Work out the finished part from the listing and answer in its coordinate system (mm). Face numbers are marked on the shaded views. A direction names the side the tool comes from. Give positions to 0.01 mm unless a question says otherwise; leave off trailing zeros. Loops run counter-clockwise (first coordinate to the right, second up) from the corner with the lowest first, then second, coordinate; pieces in that order, holes last. Notation, with made-up numbers: (-20.5, -39) - (30.5, -39) arc R22 cw to (30.5, -31) - close; hole circle Ø2 at (61, 75.25). An arc over 180 degrees is marked (long way). Use CSV: the item, a comma, the result in double quotes.
from build123d import *

# Parameters (mm, degrees)
F0_W     = 10
F0_H     = 10
F0_R     = 1.65
F1_DEPTH = 6
F0_R_2   = 4.65
F2_DEPTH = 2
F3_SIZE  = 2


with BuildPart() as f1:
    # F0 (on Top) → F1 (new body)
    with BuildSketch(Plane.XY):
        with Locations((0, 7.5)):
            Rectangle(F0_W, F0_H)
        with Locations((0, 7.5)):
            Circle(F0_R, mode=Mode.SUBTRACT)
    extrude(amount=F1_DEPTH)



with BuildPart() as f1b:
    # F0 (on Top) → F1, piece 2 (new body)
    with BuildSketch(Plane.XY):
        with Locations((0, -7.5)):
            Rectangle(F0_W, F0_H)
        with Locations((0, -7.5)):
            Circle(F0_R, mode=Mode.SUBTRACT)
    extrude(amount=F1_DEPTH)


with BuildPart() as f1_1:
    add(f1.part)

    add(f1b.part)  # F2 merges F1b
    # F0 (on Top) → F2 (join)
    with BuildSketch(Plane.XY):
        with BuildLine():
            Line((20, 25), (-20, 25))
            ThreePointArc((-20, 25), (-23.5355339059, 23.5355339059), (-25, 20))
            Line((-25, 20), (-25, -20))
            ThreePointArc((-25, -20), (-23.5355339059, -23.5355339059), (-20, -25))
            Line((-20, -25), (20, -25))
            ThreePointArc((20, -25), (23.5355339059, -23.5355339059), (25, -20))
            Line((25, -20), (25, 20))
            ThreePointArc((25, 20), (23.5355339059, 23.5355339059), (20, 25))
        make_face()
        with Locations((-17.9289321881, -17.9289321881)):
            Circle(F0_R_2, mode=Mode.SUBTRACT)
        with Locations((17.9289321881, -17.9289321881)):
            Circle(F0_R_2, mode=Mode.SUBTRACT)
        with Locations((0, -7.5)):
            Rectangle(F0_W, F0_H, mode=Mode.SUBTRACT)
        with Locations((-17.9289321881, 17.9289321881)):
            Circle(F0_R_2, mode=Mode.SUBTRACT)
        with Locations((0, 7.5)):
            Rectangle(F0_W, F0_H, mode=Mode.SUBTRACT)
        with Locations((17.9289321881, 17.9289321881)):
            Circle(F0_R_2, mode=Mode.SUBTRACT)
    extrude(amount=F2_DEPTH)

    # F3
    f3_edges = [f1_1.edges().sort_by_distance(p)[0] for p in [
        (0, -12.5, 2),
        (5, -7.5, 2),
        (5, 7.5, 2),
        (0, 2.5, 2),
        (0, -2.5, 2),
        (0, 12.5, 2),
        (-5, 7.5, 2),
        (-5, -7.5, 2),
    ]]
    chamfer(f3_edges, length=F3_SIZE)


solid = f1_1.part
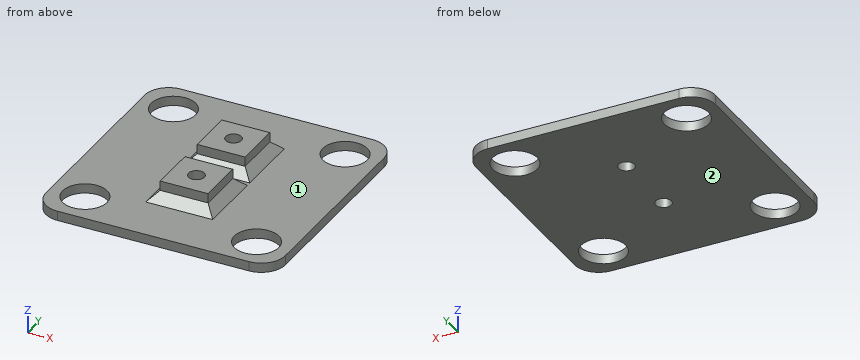
Item 1: For the marked faces 1 and 2, determine the directions among +Z, -Z, +X, -X, +Y, -Y from which every point of the face is accessible in a straight line to the end or side of a thin tool.
Determined:
face 1,"+Z"
face 2,"-Z, +X, -X, +Y, -Y"
Item 2: A cutting plane is placed at B-B on y = 7.5. Determine the outline of the cut face in (x, z), and give its area (3 significant figures).
Determined:
outline,"(-25, 0) - (-1.65, 0) - (-1.65, 6) - (-5, 6) - (-5, 4) - (-7, 2) - (-25, 2) - close; (1.65, 0) - (25, 0) - (25, 2) - (7, 2) - (5, 4) - (5, 6) - (1.65, 6) - close"
area,"124 mm²"
Item 3: Find the intervals of material crossed by line 1 (Y direction, x = 18, z = 0.75); line 2 (Y direction, x = 0, z = 1.4), in increasing order.
Determined:
line 1,"y = -25 to -22.58, -13.28 to 13.28, 22.58 to 25"
line 2,"y = -25 to -9.15, -5.85 to 5.85, 9.15 to 25"
Item 4: Given P1, Ø1.6, axis at y = -8.5, z = 5.5, coming from the +X side; P2, Ø5.5, axis at x = -17.93, y = 17.93, coming from the +Z side; P3, Ø0.6, axis at y = -9.5, z = 4.5, coming from the -X side; P4, Ø2, axis at x = 1, z = 5.5, coming from the +Y side, each flat-ended and moving along its own axis, determine where each tip first touches the part or whether it passes through.
Determined:
P1,"stops at x = 5"
P2,"passes through"
P3,"stops at x = -5"
P4,"stops at y = 12.5"
Item 5: A cutting plane is placed at C-C on x = 0. Determine the outline of the cut face in (y, z).
Determined:
outline,"(-25, 0) - (-9.15, 0) - (-9.15, 6) - (-12.5, 6) - (-12.5, 4) - (-14.5, 2) - (-25, 2) - close; (-5.85, 0) - (5.85, 0) - (5.85, 6) - (2.5, 6) - (2.5, 4) - (0.5, 2) - (-0.5, 2) - (-2.5, 4) - (-2.5, 6) - (-5.85, 6) - close; (9.15, 0) - (25, 0) - (25, 2) - (14.5, 2) - (12.5, 4) - (12.5, 6) - (9.15, 6) - close"
Item 6: A cutting plane is placed at D-D on z = 0.95. Determine the outline of the cut face in (x, y), and give its area (3 significant figures).
Determined:
outline,"(-25, -20) arc R5 ccw to (-20, -25) - (20, -25) arc R5 ccw to (25, -20) - (25, 20) arc R5 ccw to (20, 25) - (-20, 25) arc R5 ccw to (-25, 20) - close; hole circle Ø9.3 at (-17.93, -17.93); hole circle Ø9.3 at (-17.93, 17.93); hole circle Ø3.3 at (0, -7.5); hole circle Ø3.3 at (0, 7.5); hole circle Ø9.3 at (17.93, -17.93); hole circle Ø9.3 at (17.93, 17.93)"
area,"2,190 mm²"
Item 7: A cutting plane is placed at A-A on z = 4.65. Determine the outline of the cut face in (x, y).
Determined:
outline,"(-5, -12.5) - (5, -12.5) - (5, -2.5) - (-5, -2.5) - close; (-5, 2.5) - (5, 2.5) - (5, 12.5) - (-5, 12.5) - close; hole circle Ø3.3 at (0, -7.5); hole circle Ø3.3 at (0, 7.5)"
